```python
from build123d import *

# Parameters (mm, degrees)
F0_W     = 124
F0_H     = 124
F1_DEPTH = 7
F2_W     = 120.5
F2_H     = 120.5
F3_DEPTH = 4.5
F4_R     = 5.303301
F5_DEPTH = 7.001


with BuildPart() as f1:
    # F0 (on Top) → F1 (new body)
    with BuildSketch(Plane.XY):
        Rectangle(F0_W, F0_H)
    extrude(amount=F1_DEPTH)

    # F2 (on face) → F3 (cut)
    with BuildSketch(Plane.XY.offset(7)):
        Rectangle(F2_W, F2_H)
    extrude(amount=-F3_DEPTH, mode=Mode.SUBTRACT)

    # F4 (on face) → F5 (cut, through all)
    with BuildSketch(Plane(origin=(0, 0, 0), x_dir=(1, 0, 0), z_dir=(0, 0, -1))):
        with Locations((-36.093753, 44.531252)):
            Circle(F4_R)
    extrude(amount=-F5_DEPTH, mode=Mode.SUBTRACT)


solid = f1.part
```
Build history of the part. All positions in model axes, mm. A direction names the side the tool comes from. Give positions to 0.01 mm unless a question says otherwise; leave off trailing zeros. Loops run counter-clockwise (first coordinate to the right, second up) from the corner with the lowest first, then second, coordinate; pieces in that order, holes last.
Item 1: Flat gauge pin, fed straight in: pin 1 (12 mm diameter, centred on x = -36.09, y = -44.53, fed in from +Z). Where does the tip first touch, or does it go through?
Answers follow:
pin 1: stops at z = 2.5
Item 2: Pull direction X, two halves, no side cores. Call faces 1 (the face through (-1, 60.25, 5)), 2 (the face through (-62, -1, 3)), 3 (the face through (-1, 1, 0)): released by +X, released by -X, zero draft, split by the parting line, or undercut.
Answers follow:
face 1: undercut
face 2: released by -X
face 3: zero draft
Item 3: Slice it at B-B, the plane x = 33. List the corners of the cut face in (y, z), and give its area (3 significant figures).
Answers follow:
outline: (-62, 0) - (62, 0) - (62, 7) - (60.25, 7) - (60.25, 2.5) - (-60.25, 2.5) - (-60.25, 7) - (-62, 7) - close
area: 326 mm2
Item 4: Drill centre lines: line 1 (X direction, y = -12, z = 3.25); line 2 (Z direction, x = -55, y = -49). Where is each one in solid material? Low to high.
Answers follow:
line 1: x = -62 to -60.25, 60.25 to 62
line 2: z = 0 to 2.5
Item 5: Slice it at A-A, the plane z = 5.5. List the corners of the cut face in (x, y), and give its area (3 significant figures).
Answers follow:
outline: (-62, -62) - (62, -62) - (62, 62) - (-62, 62) - close; hole (-60.25, -60.25) - (60.25, -60.25) - (60.25, 60.25) - (-60.25, 60.25) - close
area: 856 mm2
Item 6: Which spindle directions (+Z, -Z, +X, -X, +Y, -Y) get a long thin tool onto all of the face, cutting with end or side? Do faces 4 (the face through (-36.78, -49.79, 1.23)), 5 (the face through (60.25, -1, 5)). Say none if no direction does.
Answers follow:
face 4: +Z, -Z
face 5: +Z
